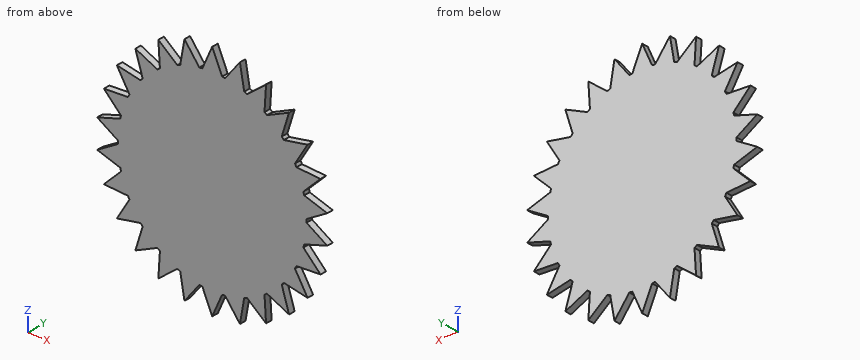
from build123d import *

# Parameters (mm, degrees)
F1_DEPTH = 2.54


with BuildPart() as f1:
    # F0 (on Front) → F1 (new body)
    with BuildSketch(Plane.XZ):
        with BuildLine():
            ThreePointArc((37.16459, -0.605521), (37.16829, -0.302771), (37.169523, 0))
            ThreePointArc((37.169523, 0), (37.16829, 0.302771), (37.16459, 0.605521))
            ThreePointArc((37.16459, 0.605521), (36.898515, 4.480291), (36.229566, 8.306143))
            ThreePointArc((36.229566, 8.306143), (36.089444, 8.895249), (35.939744, 9.481994))
            ThreePointArc((35.939744, 9.481994), (34.754108, 13.180495), (33.18901, 16.735084))
            ThreePointArc((33.18901, 16.735084), (32.911978, 17.273539), (32.626211, 17.807409))
            ThreePointArc((32.626211, 17.807409), (30.589918, 21.114696), (28.21963, 24.191443))
            ThreePointArc((28.21963, 24.191443), (27.821787, 24.647953), (27.416561, 25.097921))
            ThreePointArc((27.416561, 25.097921), (24.647953, 27.821787), (21.610228, 30.241883))
            ThreePointArc((21.610228, 30.241883), (21.114696, 30.589918), (20.61356, 30.929833))
            ThreePointArc((20.61356, 30.929833), (17.273539, 32.911978), (13.744917, 34.534775))
            ThreePointArc((13.744917, 34.534775), (13.180495, 34.754108), (12.612573, 34.964216))
            ThreePointArc((12.612573, 34.964216), (8.895249, 36.089444), (5.080802, 36.820631))
            ThreePointArc((5.080802, 36.820631), (4.480291, 36.898515), (3.87859, 36.966606))
            ThreePointArc((3.87859, 36.966606), (0, 37.169523), (-3.87859, 36.966606))
            ThreePointArc((-3.87859, 36.966606), (-4.480291, 36.898515), (-5.080802, 36.820631))
            ThreePointArc((-5.080802, 36.820631), (-8.895249, 36.089444), (-12.612573, 34.964216))
            ThreePointArc((-12.612573, 34.964216), (-13.180495, 34.754108), (-13.744917, 34.534775))
            ThreePointArc((-13.744917, 34.534775), (-17.273539, 32.911978), (-20.61356, 30.929833))
            ThreePointArc((-20.61356, 30.929833), (-21.114696, 30.589918), (-21.610228, 30.241883))
            ThreePointArc((-21.610228, 30.241883), (-24.647953, 27.821787), (-27.416561, 25.097921))
            ThreePointArc((-27.416561, 25.097921), (-27.821787, 24.647953), (-28.21963, 24.191443))
            ThreePointArc((-28.21963, 24.191443), (-30.589918, 21.114696), (-32.626211, 17.807409))
            ThreePointArc((-32.626211, 17.807409), (-32.911978, 17.273539), (-33.18901, 16.735084))
            ThreePointArc((-33.18901, 16.735084), (-34.754108, 13.180495), (-35.939744, 9.481994))
            ThreePointArc((-35.939744, 9.481994), (-36.089444, 8.895249), (-36.229566, 8.306143))
            ThreePointArc((-36.229566, 8.306143), (-36.898515, 4.480291), (-37.16459, 0.605521))
            ThreePointArc((-37.16459, 0.605521), (-37.169523, 0), (-37.16459, -0.605521))
            ThreePointArc((-37.16459, -0.605521), (-36.898515, -4.480291), (-36.229566, -8.306143))
            ThreePointArc((-36.229566, -8.306143), (-36.089444, -8.895249), (-35.939744, -9.481994))
            ThreePointArc((-35.939744, -9.481994), (-34.754108, -13.180495), (-33.18901, -16.735084))
            ThreePointArc((-33.18901, -16.735084), (-32.911978, -17.273539), (-32.626211, -17.807409))
            ThreePointArc((-32.626211, -17.807409), (-30.589918, -21.114696), (-28.21963, -24.191443))
            ThreePointArc((-28.21963, -24.191443), (-27.821787, -24.647953), (-27.416561, -25.097921))
            ThreePointArc((-27.416561, -25.097921), (-24.647953, -27.821787), (-21.610228, -30.241883))
            ThreePointArc((-21.610228, -30.241883), (-21.114696, -30.589918), (-20.61356, -30.929833))
            ThreePointArc((-20.61356, -30.929833), (-17.273539, -32.911978), (-13.744917, -34.534775))
            ThreePointArc((-13.744917, -34.534775), (-13.180495, -34.754108), (-12.612573, -34.964216))
            ThreePointArc((-12.612573, -34.964216), (-8.895249, -36.089444), (-5.080802, -36.820631))
            ThreePointArc((-5.080802, -36.820631), (-4.480291, -36.898515), (-3.87859, -36.966606))
            ThreePointArc((-3.87859, -36.966606), (0, -37.169523), (3.87859, -36.966606))
            ThreePointArc((3.87859, -36.966606), (4.480291, -36.898515), (5.080802, -36.820631))
            ThreePointArc((5.080802, -36.820631), (8.895249, -36.089444), (12.612573, -34.964216))
            ThreePointArc((12.612573, -34.964216), (13.180495, -34.754108), (13.744917, -34.534775))
            ThreePointArc((13.744917, -34.534775), (17.273539, -32.911978), (20.61356, -30.929833))
            ThreePointArc((20.61356, -30.929833), (21.114696, -30.589918), (21.610228, -30.241883))
            ThreePointArc((21.610228, -30.241883), (24.647953, -27.821787), (27.416561, -25.097921))
            ThreePointArc((27.416561, -25.097921), (27.821787, -24.647953), (28.21963, -24.191443))
            ThreePointArc((28.21963, -24.191443), (30.589918, -21.114696), (32.626211, -17.807409))
            ThreePointArc((32.626211, -17.807409), (32.911978, -17.273539), (33.18901, -16.735084))
            ThreePointArc((33.18901, -16.735084), (34.754108, -13.180495), (35.939744, -9.481994))
            ThreePointArc((35.939744, -9.481994), (36.089444, -8.895249), (36.229566, -8.306143))
            ThreePointArc((36.229566, -8.306143), (36.898515, -4.480291), (37.16459, -0.605521))
        make_face()
        with BuildLine():
            ThreePointArc((36.229566, 8.306143), (36.898515, 4.480291), (37.16459, 0.605521))
            Line((37.16459, 0.605521), (45.350049, 5.506493))
            Line((45.350049, 5.506493), (36.229566, 8.306143))
        make_face()
        with BuildLine():
            Line((45.350049, -5.506493), (37.16459, -0.605521))
            ThreePointArc((37.16459, -0.605521), (36.898515, -4.480291), (36.229566, -8.306143))
            Line((36.229566, -8.306143), (45.350049, -5.506493))
        make_face()
        with BuildLine():
            ThreePointArc((33.18901, 16.735084), (34.754108, 13.180495), (35.939744, 9.481994))
            Line((35.939744, 9.481994), (42.714469, 16.199461))
            Line((42.714469, 16.199461), (33.18901, 16.735084))
        make_face()
        with BuildLine():
            Line((42.714469, -16.199461), (35.939744, -9.481994))
            ThreePointArc((35.939744, -9.481994), (34.754108, -13.180495), (33.18901, -16.735084))
            Line((33.18901, -16.735084), (42.714469, -16.199461))
        make_face()
        with BuildLine():
            ThreePointArc((28.21963, 24.191443), (30.589918, 21.114696), (32.626211, 17.807409))
            Line((32.626211, 17.807409), (37.596479, 25.950976))
            Line((37.596479, 25.950976), (28.21963, 24.191443))
        make_face()
        with BuildLine():
            Line((37.596479, -25.950976), (32.626211, -17.807409))
            ThreePointArc((32.626211, -17.807409), (30.589918, -21.114696), (28.21963, -24.191443))
            Line((28.21963, -24.191443), (37.596479, -25.950976))
        make_face()
        with BuildLine():
            ThreePointArc((21.610228, 30.241883), (24.647953, 27.821787), (27.416561, 25.097921))
            Line((27.416561, 25.097921), (30.293519, 34.194314))
            Line((30.293519, 34.194314), (21.610228, 30.241883))
        make_face()
        with BuildLine():
            Line((30.293519, -34.194314), (27.416561, -25.097921))
            ThreePointArc((27.416561, -25.097921), (24.647953, -27.821787), (21.610228, -30.241883))
            Line((21.610228, -30.241883), (30.293519, -34.194314))
        make_face()
        with BuildLine():
            ThreePointArc((13.744917, 34.534775), (17.273539, 32.911978), (20.61356, 30.929833))
            Line((20.61356, 30.929833), (21.230009, 40.450403))
            Line((21.230009, 40.450403), (13.744917, 34.534775))
        make_face()
        with BuildLine():
            Line((21.230009, -40.450403), (20.61356, -30.929833))
            ThreePointArc((20.61356, -30.929833), (17.273539, -32.911978), (13.744917, -34.534775))
            Line((13.744917, -34.534775), (21.230009, -40.450403))
        make_face()
        with BuildLine():
            ThreePointArc((5.080802, 36.820631), (8.895249, 36.089444), (12.612573, 34.964216))
            Line((12.612573, 34.964216), (10.932689, 44.355662))
            Line((10.932689, 44.355662), (5.080802, 36.820631))
        make_face()
        with BuildLine():
            Line((10.932689, -44.355662), (12.612573, -34.964216))
            ThreePointArc((12.612573, -34.964216), (8.895249, -36.089444), (5.080802, -36.820631))
            Line((5.080802, -36.820631), (10.932689, -44.355662))
        make_face()
        with BuildLine():
            ThreePointArc((-3.87859, 36.966606), (0, 37.169523), (3.87859, 36.966606))
            Line((3.87859, 36.966606), (0, 45.683131))
            Line((0, 45.683131), (-3.87859, 36.966606))
        make_face()
        with BuildLine():
            Line((0, -45.683131), (3.87859, -36.966606))
            ThreePointArc((3.87859, -36.966606), (0, -37.169523), (-3.87859, -36.966606))
            Line((-3.87859, -36.966606), (0, -45.683131))
        make_face()
        with BuildLine():
            ThreePointArc((-12.612573, 34.964216), (-8.895249, 36.089444), (-5.080802, 36.820631))
            Line((-5.080802, 36.820631), (-10.932689, 44.355662))
            Line((-10.932689, 44.355662), (-12.612573, 34.964216))
        make_face()
        with BuildLine():
            Line((-10.932689, -44.355662), (-5.080802, -36.820631))
            ThreePointArc((-5.080802, -36.820631), (-8.895249, -36.089444), (-12.612573, -34.964216))
            Line((-12.612573, -34.964216), (-10.932689, -44.355662))
        make_face()
        with BuildLine():
            ThreePointArc((-20.61356, 30.929833), (-17.273539, 32.911978), (-13.744917, 34.534775))
            Line((-13.744917, 34.534775), (-21.230009, 40.450403))
            Line((-21.230009, 40.450403), (-20.61356, 30.929833))
        make_face()
        with BuildLine():
            Line((-21.230009, -40.450403), (-13.744917, -34.534775))
            ThreePointArc((-13.744917, -34.534775), (-17.273539, -32.911978), (-20.61356, -30.929833))
            Line((-20.61356, -30.929833), (-21.230009, -40.450403))
        make_face()
        with BuildLine():
            ThreePointArc((-27.416561, 25.097921), (-24.647953, 27.821787), (-21.610228, 30.241883))
            Line((-21.610228, 30.241883), (-30.293519, 34.194314))
            Line((-30.293519, 34.194314), (-27.416561, 25.097921))
        make_face()
        with BuildLine():
            Line((-30.293519, -34.194314), (-21.610228, -30.241883))
            ThreePointArc((-21.610228, -30.241883), (-24.647953, -27.821787), (-27.416561, -25.097921))
            Line((-27.416561, -25.097921), (-30.293519, -34.194314))
        make_face()
        with BuildLine():
            ThreePointArc((-32.626211, 17.807409), (-30.589918, 21.114696), (-28.21963, 24.191443))
            Line((-28.21963, 24.191443), (-37.596479, 25.950976))
            Line((-37.596479, 25.950976), (-32.626211, 17.807409))
        make_face()
        with BuildLine():
            Line((-37.596479, -25.950976), (-28.21963, -24.191443))
            ThreePointArc((-28.21963, -24.191443), (-30.589918, -21.114696), (-32.626211, -17.807409))
            Line((-32.626211, -17.807409), (-37.596479, -25.950976))
        make_face()
        with BuildLine():
            ThreePointArc((-35.939744, 9.481994), (-34.754108, 13.180495), (-33.18901, 16.735084))
            Line((-33.18901, 16.735084), (-42.714469, 16.199461))
            Line((-42.714469, 16.199461), (-35.939744, 9.481994))
        make_face()
        with BuildLine():
            Line((-42.714469, -16.199461), (-33.18901, -16.735084))
            ThreePointArc((-33.18901, -16.735084), (-34.754108, -13.180495), (-35.939744, -9.481994))
            Line((-35.939744, -9.481994), (-42.714469, -16.199461))
        make_face()
        with BuildLine():
            ThreePointArc((-37.16459, 0.605521), (-36.898515, 4.480291), (-36.229566, 8.306143))
            Line((-36.229566, 8.306143), (-45.350049, 5.506493))
            Line((-45.350049, 5.506493), (-37.16459, 0.605521))
        make_face()
        with BuildLine():
            Line((-45.350049, -5.506493), (-36.229566, -8.306143))
            ThreePointArc((-36.229566, -8.306143), (-36.898515, -4.480291), (-37.16459, -0.605521))
            Line((-37.16459, -0.605521), (-45.350049, -5.506493))
        make_face()
    extrude(amount=F1_DEPTH)


solid = f1.part
The model under review builds one solid part; all positions refer to its coordinate system, in mm. Coordinates: 2 decimals unless noted, no trailing zeros. Loops run counter-clockwise (first coordinate to the right, second up) from the corner with the lowest first, then second, coordinate; pieces in that order, holes last. Notation, with made-up numbers: M -19.5,76 L 10.5,76 A15 cw 10.5,89 Z; hole C 71,-22.75 d5. An arc over 180 degrees is marked long. Put each result on its own line as item: value. Start each with the question number.
Q1. Add section A-A (x = -39.5). Write out the cut boundary in (y, z).
Q2. Add section C-C (z = 11). Write out the cut boundary in (x, y), and give its area (3 significant figures).
Q3. Wall thickness on line 1 (X direction, y = -0.65, z = -30.5); line 2 (X direction, y = -1.55, z = 39); line 3 (Z direction, x = 21.5, y = -1.3): over which ranges is each line inside the solid? List them lowest first.
Q4. Clearance check with a flat-ended pin moving along its axis: pin 1 (1.5 mm diameter, centred on y = -2, z = 11, fed in from -X). State where the tip first meets the part, or that it passes through.
Q5. Add section B-B (x = 31.5). Write out the cut boundary in (y, z), and give its area (3 significant figures).
Answers:
1. outline: M -2.54,-16.38 L 0,-16.38 L 0,-13.01 L -2.54,-13.01 Z; M -2.54,-7.3 L 0,-7.3 L 0,-2 L -2.54,-2 Z; M -2.54,2 L 0,2 L 0,7.3 L -2.54,7.3 Z; M -2.54,13.01 L 0,13.01 L 0,16.38 L -2.54,16.38 Z
2. outline: M -37.47,-2.54 L 37.47,-2.54 L 37.47,0 L -37.47,0 Z
2. area: 190 mm^2
3. line 1: x = -29.13 to -22.18, -21.24 to 21.24, 22.18 to 29.13
3. line 2: x = -21.14 to -19.39, -11.89 to -6.77, -2.97 to 2.97, 6.77 to 11.89, 19.39 to 21.14
3. line 3: z = -30.32 to 30.32
4. pin 1: stops at x = -38.23
5. outline: M -2.54,-24.81 L 0,-24.81 L 0,24.81 L -2.54,24.81 Z
5. area: 126 mm^2
